CAD build for the part. Positions are in the model's coordinates, mm. A direction names the side the tool comes from. Coordinates: 2 decimals unless noted, no trailing zeros. Loops run counter-clockwise (first coordinate to the right, second up) from the corner with the lowest first, then second, coordinate; pieces in that order, holes last.
1) Two-plate mould, pull along X, no slides. Class faces 1 (the flat face through (0, 18, -37)), 2 (the cylindrical face through (9.273, -14.545, -22.185)), 3 (the cylindrical face through (-8.856, -12.41, 22.521)): +X half, -X half, draft (parallel to the pull), parting line (faces both ways), or undercut.
2) Saw through at D-D, the plane x = 0. Write the cut outline in (y, z), and give its area (3 significant figures).
3) Which spindle directions (+Z, -Z, +X, -X, +Y, -Y) get a long thin tool onto all of the face, cutting with end or side? Do faces 4 (the flat face through (-16, 0, 21)), 5 (the flat face through (7.5, 18, -41)), 6 (the flat face through (0, 9.5, 39)). Say none if no direction does.
4) Pin check, flat tips, straight feed: pin 1 Ø8 at (y, z) = (2, -24) entering from -X; pin 2 Ø3 at (x, z) = (-14.5, -10.5) entering from +Y; pin 3 Ø2 at (x, z) = (1, 2) entering from +Y. Stop position of each tip, or through.
5) Saw through at A-A, the plane x = 11.5. Write the cut outline in (y, z), and give its area (3 significant figures).
6) Wall check: line 1 along Y through (x, z) = (7.75, 23.05); line 2 along Z through (x, y) = (12, -3); line 3 along Z through (x, y) = (1.5, 10). Give the ranges that are in metal, low to high.
7) Saw through at B-B, the plane y = -16. Write the cut outline in (x, z).
8) Saw through at C-C, the plane z = 17. Write the cut outline in (x, y), and give its area (3 significant figures).
```python
from build123d import *

# Parameters (mm, degrees)
SKETCH1_R           = 18.5
BOSS_EXTRUDE1_DEPTH = 24
SKETCH2_R           = 17.25
BOSS_EXTRUDE2_DEPTH = 45
SKETCH3_R           = 6
BOSS_EXTRUDE3_DEPTH = 6
SKETCH4_R           = 3
BOSS_EXTRUDE4_DEPTH = 15
CUT_EXTRUDE1_START  = -12
CUT_EXTRUDE1_DEPTH  = 12
SKETCH6_R           = 1.5
CUT_EXTRUDE2_DEPTH  = 3
SKETCH7_W           = 15
SKETCH7_H           = 8
BOSS_EXTRUDE5_DEPTH = 20


with BuildPart() as part:
    # Sketch1 → Boss-Extrude1 (new body)
    with BuildSketch(Plane.XY):
        Circle(SKETCH1_R)
    extrude(amount=BOSS_EXTRUDE1_DEPTH)

    # Sketch2 → Boss-Extrude2 (add)
    with BuildSketch(Plane(origin=(0, 0, 0), x_dir=(-1, 0, 0), z_dir=(0, 0, -1))):
        with Locations(Location((0, 0, 0), (0, 0, 180))):
            Circle(SKETCH2_R)
    extrude(amount=BOSS_EXTRUDE2_DEPTH)

    # Sketch3 → Boss-Extrude3 (add)
    with BuildSketch(Plane.XY.offset(24)):
        with Locations((0, 7)):
            Circle(SKETCH3_R)
    extrude(amount=BOSS_EXTRUDE3_DEPTH)

    # Sketch4 → Boss-Extrude4 (add)
    with BuildSketch(Plane.XY.offset(30)):
        with Locations((0, 7)):
            Circle(SKETCH4_R)
    extrude(amount=BOSS_EXTRUDE4_DEPTH)

    # Sketch5 → Cut-Extrude1 (cut)
    with BuildSketch(Plane.XY.offset(45).offset(CUT_EXTRUDE1_START)):
        with BuildLine():
            ThreePointArc((1.658312395, 9.5), (0, 10), (-1.658312395, 9.5))
            Line((-1.658312395, 9.5), (0, 9.5))
            Line((0, 9.5), (1.658312395, 9.5))
        make_face()
    extrude(amount=CUT_EXTRUDE1_DEPTH, mode=Mode.SUBTRACT)

    # Sketch6 → Cut-Extrude2 (cut)
    with BuildSketch(Plane.XY.offset(24)):
        with Locations((7.75, 13.423393759)):
            Circle(SKETCH6_R)
        with Locations((15.5, 0)):
            Circle(SKETCH6_R)
        with Locations((7.75, -13.423393759)):
            Circle(SKETCH6_R)
        with Locations((-7.75, -13.423393759)):
            Circle(SKETCH6_R)
        with Locations((-15.5, 0)):
            Circle(SKETCH6_R)
        with Locations((-7.75, 13.423393759)):
            Circle(SKETCH6_R)
    extrude(amount=-CUT_EXTRUDE2_DEPTH, mode=Mode.SUBTRACT)

    # Sketch7 → Boss-Extrude5 (add)
    with BuildSketch(Plane(origin=(0, 0, 0), x_dir=(1, 0, 0), z_dir=(0, 1, 0))):
        with Locations((0, 41)):
            Rectangle(SKETCH7_W, SKETCH7_H)
    extrude(amount=BOSS_EXTRUDE5_DEPTH)


solid = part.part
```
Data:
1. face 1: draft
1. face 2: parting line
1. face 3: undercut
2. outline: (-18.5, 0) - (-17.25, 0) - (-17.25, -45) - (20, -45) - (20, -37) - (17.25, -37) - (17.25, 0) - (18.5, 0) - (18.5, 24) - (13, 24) - (13, 30) - (10, 30) - (10, 33) - (9.5, 33) - (9.5, 45) - (4, 45) - (4, 30) - (1, 30) - (1, 24) - (-18.5, 24) - close
2. area: 2,620 mm2
3. face 4: +Z
3. face 5: -Z, +X, +Y
3. face 6: +Z, +X, -X, +Y
4. pin 1: stops at x = -17.25
4. pin 2: stops at y = 11.34
4. pin 3: stops at y = 18.5
5. outline: (-14.49, 0) - (-12.86, 0) - (-12.86, -45) - (12.86, -45) - (12.86, 0) - (14.49, 0) - (14.49, 24) - (-14.49, 24) - close
5. area: 1,850 mm2
6. line 1: y = -16.8 to -14.92, -11.92 to 11.92, 14.92 to 16.8
6. line 2: z = -45 to 24
6. line 3: z = -45 to 30
7. outline: (-9.29, 0) - (-6.45, 0) - (-6.45, -45) - (6.45, -45) - (6.45, 0) - (9.29, 0) - (9.29, 24) - (-9.29, 24) - close
8. outline: circle Ø37 at (0, 0)
8. area: 1,080 mm2
